Work out the finished part from the listing and answer in its coordinate system (mm). A direction names the side the tool comes from. Round coordinates to 2 decimals unless told otherwise and drop trailing zeros. Write each loop counter-clockwise with the first axis right and the second up, starting at its lowest first coordinate (ties: lowest second). Pieces come first, ordered by that corner, then holes. Notation, with made-up numbers: (4.25, -22) - (36.25, -22) arc R18 ccw to (36.25, -16) - close; hole circle Ø10 at (5, 63.25). An arc over 180 degrees is marked (long way). Answer as a JSON object with one key per item and string values.
```python
from build123d import *

# Parameters (mm, degrees)
SKETCH1_W                   = 50.8
SKETCH1_H                   = 101.6
BOSS_EXTRUDE1_DEPTH         = 9.525
F_3_0_3_DIAMETER_HOLE1_D    = 3
SKETCH4_W                   = 15.875
SKETCH4_H                   = 19.05
SKETCH4_W_2                 = 19.05
SKETCH4_H_2                 = 15.875
BOSS_EXTRUDE2_DEPTH         = 9.525
F_1_4_CLEARANCE_HOLE1_D     = 6.7564
FILLET1_R                   = 6.35
SKETCH7_W                   = 63.5
SKETCH7_H                   = 28.575
CUT_EXTRUDE1_DEPTH          = 122.89684676
F_1_4_0_25_DIAMETER_HOLE1_D = 6.35


with BuildPart() as part:
    # Sketch1 → Boss-Extrude1 (new body)
    with BuildSketch(Plane.XY):
        with Locations((25.4, 50.8)):
            Rectangle(SKETCH1_W, SKETCH1_H)
    extrude(amount=BOSS_EXTRUDE1_DEPTH)

    # Ø3.0 (3) Diameter Hole1 (through all)
    with Locations(Plane.XY.offset(9.525)):
        with Locations((12.899999981, 87.60000006), (37.900000019, 87.60000006)):
            Hole(F_3_0_3_DIAMETER_HOLE1_D / 2)

    # Sketch4 → Boss-Extrude2 (add)
    with BuildSketch(Plane.XY.offset(9.525)):
        with Locations((-7.9375, 63.5)):
            Rectangle(SKETCH4_W, SKETCH4_H)
        with Locations((58.7375, 63.5)):
            Rectangle(SKETCH4_W, SKETCH4_H)
        with Locations((25.4, -7.9375)):
            Rectangle(SKETCH4_W_2, SKETCH4_H_2)
    extrude(amount=-BOSS_EXTRUDE2_DEPTH)

    # 1/4 Clearance Hole1 (through all)
    with Locations(Plane.XY.offset(9.525)):
        with Locations((-6.35, 63.5), (57.15, 63.5), (25.4, -6.35)):
            Hole(F_1_4_CLEARANCE_HOLE1_D / 2)

    # Fillet1
    fillet1_edges = [part.edges().sort_by_distance(p)[0] for p in [
        (-15.875, 73.025, 4.7625),
        (-15.875, 53.975, 4.7625),
        (0, 53.975, 4.7625),
        (0, 73.025, 4.7625),
        (50.8, 53.975, 4.7625),
        (66.675, 53.975, 4.7625),
        (66.675, 73.025, 4.7625),
        (50.8, 73.025, 4.7625),
        (34.925, -15.875, 4.7625),
        (34.925, 0, 4.7625),
        (15.875, 0, 4.7625),
        (15.875, -15.875, 4.7625),
        (0, 101.6, 4.7625),
        (50.8, 101.6, 4.7625),
        (50.8, 0, 4.7625),
        (0, 0, 4.7625),
    ]]
    fillet(fillet1_edges, radius=FILLET1_R)

    # Sketch7 → Cut-Extrude1 (cut, through all)
    with BuildSketch(Plane.XY.offset(9.525)):
        with Locations((25.4, 87.3125)):
            Rectangle(SKETCH7_W, SKETCH7_H)
    extrude(amount=-CUT_EXTRUDE1_DEPTH, mode=Mode.SUBTRACT)

    # 1/4 (0.25) Diameter Hole1 (through all)
    with Locations(Plane.XY.offset(9.525)):
        with Locations((11.1125, 31.75), (39.6875, 31.75)):
            Hole(F_1_4_0_25_DIAMETER_HOLE1_D / 2)


solid = part.part
```
Item 1: A cutting plane is placed at B-B (x = 25.4). Write down the section's boundary in (y, z) (3 decimals).
Results found:
{"outline": "(-15.875, 0) - (-9.728, 0) - (-9.728, 9.525) - (-15.875, 9.525) - close; (-2.972, 0) - (73.025, 0) - (73.025, 9.525) - (-2.972, 9.525) - close"}
Item 2: Consider line 1 along Y through (x, z) = (25.4, 7.5) (3 decimals); line 2 along Y through (x, z) = (57.15, 2.25) (3 decimals); line 3 along X through (y, z) = (63, 8) (3 decimals). Determine where each line is inside the solid, lowest interval first.
Results found:
{"line 1": "-15.875 to -9.728, -2.972 to 73.025", "line 2": "53.975 to 60.122, 66.878 to 73.025", "line 3": "-15.875 to -9.691, -3.009 to 53.809, 60.491 to 66.675"}
Item 3: A cutting plane is placed at C-C (z = 4.75). Give the number of separate pieces and of enclosed holes in the cut face, and give its area (3 significant figures).
Results found:
{"separate pieces": "1", "enclosed holes": "5", "area": "4,410 mm²"}
Item 4: For faces 1 (the flat face through (0, 27, 5)), 2 (the flat face through (59, 53.975, 5)), 3 (the flat face through (66.675, 63, 5)), determine the directions among +Z, -Z, +X, -X, +Y, -Y from which every point of the face is accessible in a straight line to the end or side of a thin tool.
Results found:
{"face 1": "+Z, -Z, -X, -Y", "face 2": "+Z, -Z, +X, -Y", "face 3": "+Z, -Z, +X, +Y, -Y"}
Item 5: Determine the mould class of faces 4 (the cylindrical face through (48.89, 1.81, 4.83)), 5 (the flat face through (25, 73.025, 5)), 6 (the cylindrical face through (-5.62, 60.2, 4.7)) for opening direction Y: pulls with the +Y half, pulls with the -Y half, needs draft (parallel to the pull), parting line crosses it, or undercut.
Results found:
{"face 4": "pulls with the -Y half", "face 5": "pulls with the +Y half", "face 6": "undercut"}
Item 6: Each of these flat-tipped pins is pushed along its axis until it touches: P1, Ø2, axis at x = 0.5, z = 2, coming from the -Y side; P2, Ø4, axis at x = 57.15, y = 63.5, coming from the -Z side; P3, Ø1.6, axis at x = 59, z = 6, coming from the -Y side (3 decimals); P4, Ø3.5, axis at x = 8, z = 4.5, coming from the -Y side. Where does it stop, or does it pass through?
Results found:
{"P1": "y = 2.25", "P2": "through", "P3": "y = 53.975", "P4": "y = 0"}
Item 7: A cutting plane is placed at D-D (y = 31.75). Write down the section's boundary in (x, z) (1 decimal).
Results found:
{"outline": "(0, 0) - (7.9, 0) - (7.9, 9.5) - (0, 9.5) - close; (14.3, 0) - (36.5, 0) - (36.5, 9.5) - (14.3, 9.5) - close; (42.9, 0) - (50.8, 0) - (50.8, 9.5) - (42.9, 9.5) - close"}
Item 8: A cutting plane is placed at A-A (y = 63.5). Write down the section's boundary in (x, z) (3 decimals), and give its area (3 significant figures).
Results found:
{"outline": "(-15.875, 0) - (-9.728, 0) - (-9.728, 9.525) - (-15.875, 9.525) - close; (-2.972, 0) - (53.772, 0) - (53.772, 9.525) - (-2.972, 9.525) - close; (60.528, 0) - (66.675, 0) - (66.675, 9.525) - (60.528, 9.525) - close", "area": "658 mm²"}
